Work out the finished part from the listing and answer in its coordinate system (mm). A direction names the side the tool comes from. Round coordinates to 2 decimals unless told otherwise and drop trailing zeros. Loops run counter-clockwise (first coordinate to the right, second up) from the corner with the lowest first, then second, coordinate; pieces in that order, holes last. Notation, with made-up numbers: (59, -21.75) -> (109, -21.75) arc R26 cw to (109, 10.25) -> close; hole circle Ø8 at (29, -40). An arc over 180 degrees is marked (long way). Use one line per item in the form item = value.
```python
from build123d import *

# Parameters (mm, degrees)
F0_W     = 100
F0_H     = 100
F1_DEPTH = 20
F2_R     = 3.7625
F3_DEPTH = 25


with BuildPart() as f1:
    # F0 (on Top) → F1 (new body)
    with BuildSketch(Plane.XY):
        with BuildLine():
            ThreePointArc((46.9041575982, 105), (81.3172798365, 81.3172798365), (105, 46.9041575982))
            Line((105, 46.9041575982), (105, 105))
            Line((105, 105), (46.9041575982, 105))
        make_face()
        with BuildLine():
            ThreePointArc((-105, 46.9041575982), (-81.3172798365, 81.3172798365), (-46.9041575982, 105))
            Line((-46.9041575982, 105), (-105, 105))
            Line((-105, 105), (-105, 46.9041575982))
        make_face()
        with BuildLine():
            Line((-105, -105), (-46.9041575982, -105))
            ThreePointArc((-46.9041575982, -105), (-81.3172798365, -81.3172798365), (-105, -46.9041575982))
            Line((-105, -46.9041575982), (-105, -105))
        make_face()
        with BuildLine():
            Line((105, -105), (105, -46.9041575982))
            ThreePointArc((105, -46.9041575982), (81.3172798365, -81.3172798365), (46.9041575982, -105))
            Line((46.9041575982, -105), (105, -105))
        make_face()
        with BuildLine():
            Line((105, -46.9041575982), (105, 46.9041575982))
            ThreePointArc((105, 46.9041575982), (81.3172798365, 81.3172798365), (46.9041575982, 105))
            Line((46.9041575982, 105), (-46.9041575982, 105))
            ThreePointArc((-46.9041575982, 105), (-81.3172798365, 81.3172798365), (-105, 46.9041575982))
            Line((-105, 46.9041575982), (-105, -46.9041575982))
            ThreePointArc((-105, -46.9041575982), (-81.3172798365, -81.3172798365), (-46.9041575982, -105))
            Line((-46.9041575982, -105), (46.9041575982, -105))
            ThreePointArc((46.9041575982, -105), (81.3172798365, -81.3172798365), (105, -46.9041575982))
        make_face()
        Rectangle(F0_W, F0_H, mode=Mode.SUBTRACT)
    extrude(amount=F1_DEPTH)

    # F2 (on Top) → F3 (cut)
    with BuildSketch(Plane.XY):
        with Locations((-70.8591109885, 59.457853896)):
            Circle(F2_R)
        with Locations((-46.25, -80.1073498501)):
            Circle(F2_R)
    extrude(amount=F3_DEPTH, mode=Mode.SUBTRACT)


solid = f1.part
```
(1) For a pull along Y with two mould halves and no side action, classify faces 3 (the flat face through (50, -1, 10)), 4 (the flat face through (-1, -105, 10)), 5 (the flat face through (-71, 1, 20)) as +Y half, -Y half, draft (parallel to the pull), parting line (faces both ways), or undercut.
Completed:
face_3 = undercut
face_4 = -Y half
face_5 = draft
(2) Consider L1, parallel to Y at x = -46.25, z = 5; L2, parallel to X at y = 23.5, z = 10.25. Determine where each line is inside the solid, lowest interval first.
Completed:
L1 = -105 to -83.87, -76.34 to -50, 50 to 105
L2 = -105 to -50, 50 to 105
(3) Find section A-A, the plane x = -46.25. Write down the section's boundary in (y, z).
Completed:
outline = (-105, 0) -> (-83.87, 0) -> (-83.87, 20) -> (-105, 20) -> close; (-76.34, 0) -> (-50, 0) -> (-50, 20) -> (-76.34, 20) -> close; (50, 0) -> (105, 0) -> (105, 20) -> (50, 20) -> close
(4) Find section B-B, the plane y = -29. Write down the section's boundary in (x, z).
Completed:
outline = (-105, 0) -> (-50, 0) -> (-50, 20) -> (-105, 20) -> close; (50, 0) -> (105, 0) -> (105, 20) -> (50, 20) -> close
(5) For faces 1 (the flat face through (-1, 50, 10)), 2 (the flat face through (105, -1, 10)), determine the directions among +Z, -Z, +X, -X, +Y, -Y from which every point of the face is accessible in a straight line to the end or side of a thin tool.
Completed:
face_1 = +Z, -Z
face_2 = +Z, -Z, +X, +Y, -Y
(6) Given P1, Ø12, axis at x = -46.25, y = -80.11, coming from the -Z side, flat-ended and moving along its own axis, determine where the tip first touches the part or whether it passes through.
Completed:
P1 = 0
(7) Find section D-D, the plane z = 6. State how many separate pieces and enclosed holes the cut face has, then the cut area to 3 significant figures.
Completed:
separate_pieces = 1
enclosed_holes = 3
area = 34,000 mm2
